Geometry: final body of the model. Coordinates: model frame, mm. Face numbers are marked on the shaded views. A direction names the side the tool comes from. Give positions to 0.01 mm unless a question says otherwise; leave off trailing zeros. Loops run counter-clockwise (first coordinate to the right, second up) from the corner with the lowest first, then second, coordinate; pieces in that order, holes last. Notation, with made-up numbers: (-22.75, 19) - (30.25, 19) arc R22 ccw to (30.25, 27) - close; hole circle Ø7 at (45.5, 56). An arc over 180 degrees is marked (long way). Answer in a Markdown table with one row per item.
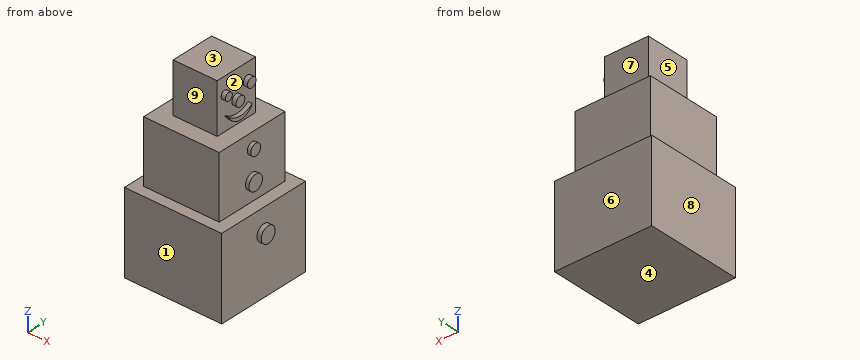
from build123d import *

# Parameters (mm, degrees)
F0_W      = 77.780351
F0_H      = 76.820102
F1_DEPTH  = 65
F2_W      = 60.396654
F2_H      = 60.396655
F3_DEPTH  = 50
F4_W      = 35.160178
F4_H      = 35.160179
F5_DEPTH  = 40
F6_R      = 3.166361
F6_R_2    = 3.894654
F6_R_3    = 4.007563
F6_R_4    = 4.561233
F6_R_5    = 6.154541
F6_R_6    = 6.407927
F7_DEPTH  = 25.4
F8_R      = 4.561233
F8_R_2    = 6.154541
F8_R_3    = 4.007563
F8_R_4    = 3.894654
F8_R_5    = 3.166361
F9_DEPTH  = 10
F10_R     = 3.166361
F10_R_2   = 4.007563
F10_R_3   = 3.894654
F11_DEPTH = 12


with BuildPart() as f1:
    # F0 (on Top) → F1 (new body)
    with BuildSketch(Plane.XY):
        with Locations((-2.563856, 10.494465)):
            Rectangle(F0_W, F0_H)
    extrude(amount=F1_DEPTH)

    # F2 (on face) → F3 (join)
    with BuildSketch(Plane.XY.offset(65)):
        with Locations((-3.268891, 10.740642)):
            Rectangle(F2_W, F2_H)
    extrude(amount=F3_DEPTH)

    # F4 (on face) → F5 (join)
    with BuildSketch(Plane.XY.offset(115)):
        with Locations((-3.268891, 10.740642)):
            Rectangle(F4_W, F4_H)
    extrude(amount=F5_DEPTH)

    # F6 (on face) → F7 (join)
    with BuildSketch(Plane.YZ.offset(14.311198)):
        with Locations((0, 141.694024)):
            Circle(F6_R)
        with Locations((20.969419, 141.694024)):
            Circle(F6_R_2)
        with Locations((10.578918, 133.192703)):
            Circle(F6_R_3)
        with BuildLine():
            ThreePointArc((21.463975, 126.287654), (10.662218, 122.715489), (0, 126.6848))
            ThreePointArc((0, 126.6848), (10.609036, 119.841253), (21.463975, 126.287654))
        make_face()
        with Locations((10.830865, 103.396073)):
            Circle(F6_R_4)
        with Locations((10.830865, 79.781286)):
            Circle(F6_R_5)
        with Locations((10.830865, 46.720583)):
            Circle(F6_R_6)
    extrude(amount=F7_DEPTH)

    # F8 (on face) → F9 (cut)
    with BuildSketch(Plane.YZ.offset(39.711198)):
        with Locations((10.830865, 103.396073)):
            Circle(F8_R)
        with BuildLine():
            ThreePointArc((0, 126.6848), (10.609036, 119.841253), (21.463975, 126.287654))
            ThreePointArc((21.463975, 126.287654), (10.662218, 122.715489), (0, 126.6848))
        make_face()
        with Locations((10.830865, 79.781286)):
            Circle(F8_R_2)
        with Locations((10.578918, 133.192703)):
            Circle(F8_R_3)
        with Locations((20.969419, 141.694024)):
            Circle(F8_R_4)
        with Locations((0, 141.694024)):
            Circle(F8_R_5)
    extrude(amount=-F9_DEPTH, mode=Mode.SUBTRACT)

    # F10 (on face) → F11 (cut)
    with BuildSketch(Plane.YZ.offset(29.711198)):
        with Locations((0, 141.694024)):
            Circle(F10_R)
        with Locations((10.578918, 133.192703)):
            Circle(F10_R_2)
        with Locations((20.969419, 141.694024)):
            Circle(F10_R_3)
        with BuildLine():
            ThreePointArc((0, 126.6848), (10.609036, 119.841253), (21.463975, 126.287654))
            ThreePointArc((21.463975, 126.287654), (10.662218, 122.715489), (0, 126.6848))
        make_face()
    extrude(amount=-F11_DEPTH, mode=Mode.SUBTRACT)


solid = f1.part
Q1. Cut plane D-D (x = 33). Output: boundary loops of the cut face in (y, z), and give its area (3 significant figures).
Check values:
| item | result |
|---|---|
| outline | (-27.92, 0) - (48.9, 0) - (48.9, 65) - (-27.92, 65) - close |
| area | 4,990 mm² |
Q2. Reachability of the marked faces 5, 6, 7, 8 and 9 from +Z, -Z, +X, -X, +Y, -Y: full face, straight path, thin tool, end or side. Return the list, or none.
Check values:
| item | result |
|---|---|
| face 5 | +Z, -X, +Y, -Y |
| face 6 | +Z, -Z, +X, -X, +Y |
| face 7 | +Z, +X, -X, +Y |
| face 8 | +Z, -Z, -X, +Y, -Y |
| face 9 | +Z, +X, -X, -Y |
Q3. Cut plane B-B (x = -3). Output: boundary loops of the cut face in (y, z), and give its area (3 significant figures).
Check values:
| item | result |
|---|---|
| outline | (-27.92, 0) - (48.9, 0) - (48.9, 65) - (40.94, 65) - (40.94, 115) - (28.32, 115) - (28.32, 155) - (-6.84, 155) - (-6.84, 115) - (-19.46, 115) - (-19.46, 65) - (-27.92, 65) - close |
| area | 9,420 mm² |
Q4. Cut plane A-A (y = -11). Output: boundary loops of the cut face in (x, z), and give its area (3 significant figures).
Check values:
| item | result |
|---|---|
| outline | (-41.45, 0) - (36.33, 0) - (36.33, 65) - (26.93, 65) - (26.93, 115) - (-33.47, 115) - (-33.47, 65) - (-41.45, 65) - close |
| area | 8,080 mm² |
Q5. Draft query along Z for the marked faces 1, 2, 3 and 4. Return one class per face: pulls with the +Z half, pulls with the -Z half, needs draft (parallel to the pull), parting line crosses it, or undercut.
Check values:
| item | result |
|---|---|
| face 1 | needs draft |
| face 2 | undercut |
| face 3 | pulls with the +Z half |
| face 4 | pulls with the -Z half |
Q6. Cut plane C-C (z = 58). Output: boundary loops of the cut face in (x, y).
Check values:
| item | result |
|---|---|
| outline | (-41.45, -27.92) - (36.33, -27.92) - (36.33, 48.9) - (-41.45, 48.9) - close |
Q7. Material intervals for line 1 along Z through (x, y) = (10.5, 37); line 2 along X through (y, z) = (17, 92.5); line 3 along X through (y, z) = (-21, 50), sorted ascending.
Check values:
| item | result |
|---|---|
| line 1 | 0 to 115 |
| line 2 | -33.47 to 26.93 |
| line 3 | -41.45 to 36.33 |
Q8. First-contact query: pin 1 (10.5 mm diameter, centred on x = -5, z = 133.5, fed in from +Y); pin 2 (7 mm diameter, centred on y = -1, z = 141.5, fed in from +X); pin 3 (2 mm diameter, centred on y = 12, z = 96.5, fed in from -X). Flat tips, straight axial feed; report the tip coordinate or a pass-through.
Check values:
| item | result |
|---|---|
| pin 1 | y = 28.32 |
| pin 2 | x = 17.71 |
| pin 3 | x = -33.47 |
